from build123d import *

# Parameters (mm, degrees)
F0_W      = 460
F0_H      = 140
F1_DEPTH  = 50
F2_R      = 10
F3_DEPTH  = 25
F3_FACE_R = 10
F4_DEPTH  = 25
F5_R      = 10
F6_R      = 10


with BuildPart() as f1:
    # F0 (on Top) → F1 (new body)
    with BuildSketch(Plane.XY):
        with Locations((-3.7046, -2.36354)):
            Rectangle(F0_W, F0_H)
    extrude(amount=F1_DEPTH)

    # F2 (on face) → F3 (cut)
    with BuildSketch(Plane(origin=(0, 0, 0), x_dir=(1, 0, 0), z_dir=(0, 0, -1))):
        with Locations((146.342196, 0)):
            Circle(F2_R)
    extrude(amount=-F3_DEPTH, mode=Mode.SUBTRACT)

    # F3_face (on face) → F4 (cut)
    with BuildSketch(Plane(origin=(146.342196, 0, 25), x_dir=(1, 0, 0), z_dir=(0, 0, -1))):
        Circle(F3_FACE_R)
    extrude(amount=-F4_DEPTH, mode=Mode.SUBTRACT)

    # F5
    f5_edges = [f1.edges().sort_by_distance(p)[0] for p in [
        (-233.7046, -72.36354, 25),
        (-3.7046, -72.36354, 50),
        (-233.7046, -2.36354, 50),
    ]]
    fillet(f5_edges, radius=F5_R)

    # F6
    f6_edges = [f1.edges().sort_by_distance(p)[0] for p in [
        (226.2954, -72.36354, 20),
        (226.2954, 67.63646, 25),
        (1.2954, 67.63646, 50),
    ]]
    fillet(f6_edges, radius=F6_R)


solid = f1.part
Can you work these out from the model? Positions are in its coordinate system, mm. Round coordinates to 2 decimals unless told otherwise and drop trailing zeros. Loops run counter-clockwise (first coordinate to the right, second up) from the corner with the lowest first, then second, coordinate; pieces in that order, holes last. Notation, with made-up numbers: (38, -35.75) - (64, -35.75) arc R7 ccw to (64, -25.75) - close; hole circle Ø7 at (36.25, 47). An arc over 180 degrees is marked (long way). Answer in a Markdown table with one row per item. Add a question column.
Q1. I need wall thicknesses on L1, parallel to X at y = 0, z = 15; L2, parallel to Z at x = 155, y = 60; L3, parallel to X at y = -8.5, z = 30.5. Which ranges of each line are inside material? Lowest first, please.
Q2. I want a section at A-A on y = 0. List the corners of the cut face in (x, z) for me, and give its area (3 significant figures).
Q3. We'd pull the mould along X, two halves only. Please class faces 1 (the cylindrical face through (223.288, 64.785, 20.28)), 2 (the cylindrical face through (-230.85, -69.36, 20.28)), 3 (the cylindrical face through (136.35, -0.44, 24.65)), 4 (the flat face through (-7, -72.364, 20)): pulls with the +X half, pulls with the -X half, needs draft (parallel to the pull), parting line crosses it, or undercut.
Q4. For pin 1 Ø1 at (y, z) = (-43.5, 42) entering from -X; pin 2 Ø6 at (x, y) = (-91.5, 50) entering from -Z, each with a flat end and sliding along its axis, tell me the tip position at first contact or that it passes through.
A:
| question | item | result |
|---|---|---|
| 1 | L1 | -233.7 to 136.34, 156.34 to 226.3 |
| 1 | L2 | 0 to 49.72 |
| 1 | L3 | -233.7 to 141.07, 151.61 to 226.3 |
| 2 | outline | (-233.7, 0) - (136.34, 0) - (136.34, 50) - (-223.7, 50) arc R10 ccw to (-233.7, 40) - close; (156.34, 0) - (226.3, 0) - (226.3, 40) arc R10 ccw to (216.3, 50) - (156.34, 50) - close |
| 2 | area | 22,000 mm^2 |
| 3 | face 1 | pulls with the +X half |
| 3 | face 2 | pulls with the -X half |
| 3 | face 3 | undercut |
| 3 | face 4 | needs draft |
| 4 | pin 1 | x = -233.59 |
| 4 | pin 2 | z = 0 |
